Source: CAD feature listing. Evaluate the final solid. Frame: model axes, mm. Coordinates: 2 decimals unless noted, no trailing zeros. Order: outer loops, then holes, each group sorted by start corner. A loop starts at its lowest first (then second) coordinate and runs counter-clockwise, first axis right, second up. Notation, with made-up numbers: (56, 32.25) -> (97, 32.25) arc R5 ccw to (97, 40.25) -> close; hole circle Ø5 at (54, 9). An arc over 180 degrees is marked (long way). Put each result on its own line as item: value.
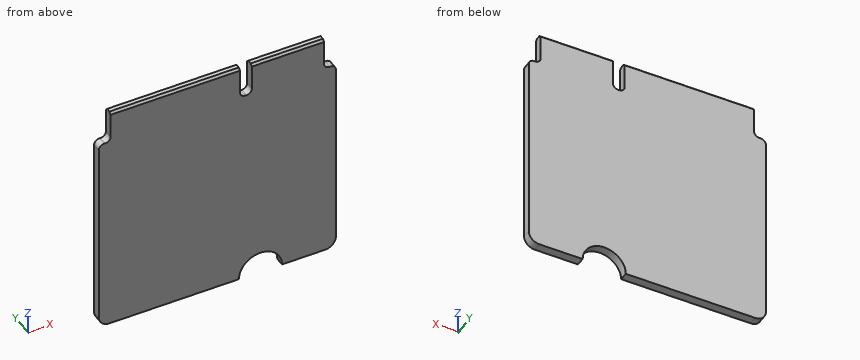
from build123d import *

# Parameters (mm, degrees)
BOSS_EXTRUDE1_DEPTH = 0.8
FILLET1_R           = 1
FILLET2_R           = 0.5
CHAMFER1_SIZE       = 0.2


with BuildPart() as part:
    # Sketch1 → Boss-Extrude1 (new body)
    with BuildSketch(Plane(origin=(0, 0, 0), x_dir=(1, 0, 0), z_dir=(0, 1, 0))):
        with BuildLine():
            Line((14.2, -22), (20.9, -22))
            Line((20.9, -22), (20.9, -19))
            Line((20.9, -19), (22, -19))
            Line((22, -19), (22, 0))
            Line((22, 0), (17, 0))
            ThreePointArc((17, 0), (15, -2), (13, 0))
            Line((13, 0), (0, 0))
            Line((0, 0), (0, -19))
            Line((0, -19), (1.1, -19))
            Line((1.1, -19), (1.1, -22))
            Line((1.1, -22), (13.1, -22))
            Line((13.1, -22), (13.1, -19))
            Line((13.1, -19), (14.2, -19))
            Line((14.2, -19), (14.2, -22))
        make_face()
    extrude(amount=BOSS_EXTRUDE1_DEPTH)

    # Fillet1
    fillet1_edges = [part.edges().sort_by_distance(p)[0] for p in [
        (0, 0.4, 0),
        (22, 0.4, 0),
    ]]
    fillet(fillet1_edges, radius=FILLET1_R)

    # Fillet2
    fillet2_edges = [part.edges().sort_by_distance(p)[0] for p in [
        (22, 0.4, 19),
        (20.9, 0.4, 19),
        (14.2, 0.4, 19),
        (13.1, 0.4, 19),
        (1.1, 0.4, 19),
        (0, 0.4, 19),
    ]]
    fillet(fillet2_edges, radius=FILLET2_R)

    # Chamfer1
    chamfer1_edges = [part.edges().sort_by_distance(p)[0] for p in [
        (17.55, 0, 22),
        (7.1, 0.8, 22),
        (7.1, 0, 22),
        (17.55, 0.8, 22),
    ]]
    chamfer(chamfer1_edges, length=CHAMFER1_SIZE)


solid = part.part
1. Cut plane A-A on y = 0.45. Output: boundary loops of the cut face in (x, z), plus the area to 3 significant figures.
Numbers:
outline: (0, 1) arc R1 ccw to (1, 0) -> (13, 0) arc R2 cw to (17, 0) -> (21, 0) arc R1 ccw to (22, 1) -> (22, 18.5) arc R0.5 ccw to (21.5, 19) -> (21.4, 19) arc R0.5 cw to (20.9, 19.5) -> (20.9, 22) -> (14.2, 22) -> (14.2, 19.5) arc R0.5 cw to (13.7, 19) -> (13.6, 19) arc R0.5 cw to (13.1, 19.5) -> (13.1, 22) -> (1.1, 22) -> (1.1, 19.5) arc R0.5 cw to (0.6, 19) -> (0.5, 19) arc R0.5 ccw to (0, 18.5) -> close
area: 467 mm2
2. Ray query, line 1 along X through (y, z) = (0.4, 19.75); line 2 along Z through (x, y) = (16, 0.4); line 3 along Z through (x, y) = (7.5, 0.7). Return the intervals inside material, ascending.
Numbers:
line 1: x = 1.1 to 13.1, 14.2 to 20.9
line 2: z = 1.73 to 22
line 3: z = 0 to 21.9
3. Cut plane B-B on x = 15. Output: boundary loops of the cut face in (y, z).
Numbers:
outline: (0, 2) -> (0.8, 2) -> (0.8, 21.8) -> (0.6, 22) -> (0.2, 22) -> (0, 21.8) -> close
